from build123d import *

# Parameters (mm, degrees)
SKETCH1_R           = 38.1
BOSS_EXTRUDE1_DEPTH = 50.8
SKETCH2_W           = 38.1
SKETCH2_H           = 12.7
SKETCH2_W_2         = 1.5875
SKETCH2_H_2         = 34.925
SKETCH4_R           = 6.35
BOSS_EXTRUDE2_DEPTH = 6.35
BOSS_EXTRUDE3_DEPTH = 9.525
FILLET1_R           = 2.54
SKETCH6_W           = 3.175
SKETCH6_H           = 12.7
CUT_EXTRUDE1_DEPTH  = 12.7
SHELL1_START        = 3.81
SHELL1_OUTLINE_R    = 22.86
SHELL1_OUTLINE_W    = 8.255
SHELL1_OUTLINE_H    = 17.78
SHELL1_DEPTH        = 42.8625
SHELL1_START_2      = 7.9375
SHELL1_2_OUTLINE_W  = 8.255
SHELL1_2_OUTLINE_H  = 17.78
SHELL1_2_DEPTH      = 38.735
SHELL1_START_3      = 58.1025
SHELL1_3_DEPTH      = 4.445
SHELL1_START_4      = 46.6725
SHELL1_4_OUTLINE_R  = 3.81
SHELL1_4_DEPTH      = 11.43
SHELL1_START_5      = -2.2225
SHELL1_6_OUTLINE_R  = 19.05
SHELL1_6_OUTLINE_W  = 8.255
SHELL1_6_OUTLINE_H  = 17.78
SHELL1_6_DEPTH      = 6.0325


with BuildPart() as part:
    # Sketch1 → Boss-Extrude1 (new body)
    with BuildSketch(Plane.XY):
        Circle(SKETCH1_R)
    extrude(amount=BOSS_EXTRUDE1_DEPTH)

    # Sketch2 → Cut-Revolve1 (revolve, cut)
    with BuildSketch(Plane(origin=(0, 0, 0), x_dir=(0, 0, -1), z_dir=(1, 0, 0))):
        with Locations((-25.4, 31.75)):
            Rectangle(SKETCH2_W, SKETCH2_H)
        with Locations((-0.79375, 17.4625)):
            Rectangle(SKETCH2_W_2, SKETCH2_H_2)
        with Locations((-50.00625, 17.4625)):
            Rectangle(SKETCH2_W_2, SKETCH2_H_2)
    revolve(axis=Axis((0, 0, 0), (0, 0, 1)), mode=Mode.SUBTRACT)

    # Sketch3 → Revolve1 (revolve)
    with BuildSketch(Plane(origin=(0, 0, 0), x_dir=(0, 0, -1), z_dir=(1, 0, 0))):
        with BuildLine():
            Line((4.7625, 19.05), (4.7625, 0))
            Line((4.7625, 0), (-1.5875, 0))
            Line((-1.5875, 0), (-1.5875, 25.4))
            Line((-1.5875, 25.4), (1.99026356, 23.575552712))
            ThreePointArc((1.99026356, 23.575552712), (4.014349425, 21.703578821), (4.7625, 19.05))
        make_face()
    revolve(axis=Axis((0, 0, -4.7625), (0, 0, 1)))

    # Sketch4 → Boss-Extrude2 (add)
    with BuildSketch(Plane.XY.offset(49.2125)):
        with Locations(Location((0, 0, 0), (0, 0, 90))):
            Circle(SKETCH4_R)
    extrude(amount=BOSS_EXTRUDE2_DEPTH)

    # Sketch5 → Boss-Extrude3 (add)
    with BuildSketch(Plane.XY.offset(55.5625)):
        with BuildLine():
            Line((-2.358330795, 25.854173013), (-11.945334146, 1.886664636))
            ThreePointArc((-11.945334146, 1.886664636), (-12.308672556, 0), (-11.945334146, -1.886664636))
            Line((-11.945334146, -1.886664636), (-2.358330795, -25.854173013))
            ThreePointArc((-2.358330795, -25.854173013), (0, -27.450840695), (2.358330795, -25.854173013))
            Line((2.358330795, -25.854173013), (11.945334146, -1.886664636))
            ThreePointArc((11.945334146, -1.886664636), (12.308672556, 0), (11.945334146, 1.886664636))
            Line((11.945334146, 1.886664636), (2.358330795, 25.854173013))
            ThreePointArc((2.358330795, 25.854173013), (0, 27.450840695), (-2.358330795, 25.854173013))
        make_face()
    extrude(amount=BOSS_EXTRUDE3_DEPTH)

    # Fillet1
    fillet1_edges = [part.edges().sort_by_distance(p)[0] for p in [
        (0, -27.450840695, 65.0875),
        (7.15183247, -13.870418824, 65.0875),
        (12.308672556, 0, 65.0875),
        (7.15183247, 13.870418824, 65.0875),
        (0, 27.450840695, 65.0875),
        (-7.15183247, 13.870418824, 65.0875),
        (-12.308672556, 0, 65.0875),
        (-7.15183247, -13.870418824, 65.0875),
    ]]
    fillet(fillet1_edges, radius=FILLET1_R)

    # Sketch6 → Cut-Extrude1 (cut)
    with BuildSketch(Plane(origin=(0, 0, -4.7625), x_dir=(-1, 0, 0), z_dir=(0, 0, -1))):
        Rectangle(SKETCH6_W, SKETCH6_H)
    extrude(amount=-CUT_EXTRUDE1_DEPTH, mode=Mode.SUBTRACT)

    # Shell1: read off the stored shape, not the designer's step
    # Shell1 outline → Shell1 (cut)
    with BuildSketch(Plane.XY.offset(SHELL1_START)):
        Circle(SHELL1_OUTLINE_R)
        Rectangle(SHELL1_OUTLINE_W, SHELL1_OUTLINE_H, mode=Mode.SUBTRACT)
    extrude(amount=SHELL1_DEPTH, mode=Mode.SUBTRACT)

    # Shell1 2 outline → Shell1 2 (cut)
    with BuildSketch(Plane.XY.offset(SHELL1_START_2)):
        Rectangle(SHELL1_2_OUTLINE_W, SHELL1_2_OUTLINE_H)
    extrude(amount=SHELL1_2_DEPTH, mode=Mode.SUBTRACT)

    # Shell1 3 outline → Shell1 3 (cut)
    with BuildSketch(Plane.XY.offset(SHELL1_START_3)):
        with BuildLine():
            Line((9.587003351, 0.943332318), (0, 24.910840695))
            Line((0, 24.910840695), (-9.587003351, 0.943332318))
            ThreePointArc((-9.587003351, 0.943332318), (-9.768672556, 0), (-9.587003351, -0.943332318))
            Line((-9.587003351, -0.943332318), (0, -24.910840695))
            Line((0, -24.910840695), (9.587003351, -0.943332318))
            ThreePointArc((9.587003351, -0.943332318), (9.768672556, 0), (9.587003351, 0.943332318))
        make_face()
    extrude(amount=SHELL1_3_DEPTH, mode=Mode.SUBTRACT)

    # Shell1 4 outline → Shell1 4 (cut)
    with BuildSketch(Plane.XY.offset(SHELL1_START_4)):
        Circle(SHELL1_4_OUTLINE_R)
    extrude(amount=SHELL1_4_DEPTH, mode=Mode.SUBTRACT)

    # Shell1 5 outline → Shell1 5 (revolve, cut)
    with BuildSketch(Plane.XZ):
        with BuildLine():
            ThreePointArc((19.05, -2.2225), (20.37678941, -1.848424713), (21.312776356, -0.83638178))
            Line((21.312776356, -0.83638178), (23.682155577, 3.81))
            Line((23.682155577, 3.81), (19.05, 3.81))
            Line((19.05, 3.81), (19.05, -2.2225))
        make_face()
    revolve(axis=Axis((0, 0, 0), (0, 0, 1)), mode=Mode.SUBTRACT)

    # Shell1 6 outline → Shell1 6 (cut)
    with BuildSketch(Plane.XY.offset(SHELL1_START_5)):
        Circle(SHELL1_6_OUTLINE_R)
        Rectangle(SHELL1_6_OUTLINE_W, SHELL1_6_OUTLINE_H, mode=Mode.SUBTRACT)
    extrude(amount=SHELL1_6_DEPTH, mode=Mode.SUBTRACT)


solid = part.part
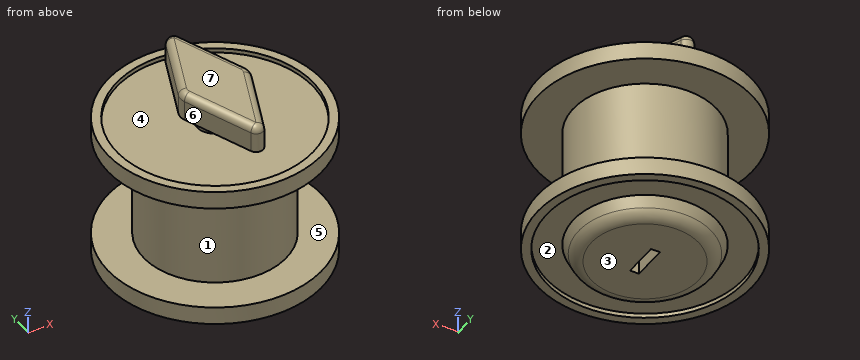
Read the model definition and answer for the solid it produces. Units are mm, in the model's axes. Face numbers are marked on the shaded views. A direction names the side the tool comes from. Coordinates: 2 decimals unless noted, no trailing zeros. Order: outer loops, then holes, each group sorted by start corner. A loop starts at its lowest first (then second) coordinate and runs counter-clockwise, first axis right, second up. Notation, with made-up numbers: (86, 11.5) -> (90, 11.5) arc R27 cw to (90, 36.5) -> close; hole circle Ø4 at (0, -39.75). An arc over 180 degrees is marked (long way). Answer as a JSON object with one key per item and string values.
1) A cutting plane is placed at C-C, the plane z = 23.5. Determine the outline of the cut face in (x, y), plus the area to 3 significant figures.
Model answer:
{"outline": "circle Ø50.8 at (0, 0); hole circle Ø45.72 at (0, 0)", "area": "385 mm²"}
2) Consider line 1 along Z through (x, y) = (5.5, -4.5); line 2 along Z through (x, y) = (-34, 10); line 3 along Z through (x, y) = (18, 2). Determine where each line is inside the solid, lowest interval first. Write a range as from..to.
Model answer:
{"line 1": "z = -4.76..-2.22, 46.67..49.21, 55.56..58.1, 62.55..65.09", "line 2": "z = 0..6.35, 44.45..50.8", "line 3": "z = -4.76..-2.22, 46.67..49.21"}
3) A cutting plane is placed at A-A, the plane y = -33. Determine the outline of the cut face in (x, z), plus the area to 3 significant figures.
Model answer:
{"outline": "(-19.04, 0) -> (-11.43, 0) -> (-11.43, 1.59) -> (11.43, 1.59) -> (11.43, 0) -> (19.04, 0) -> (19.04, 6.35) -> (-19.04, 6.35) -> close; (-19.04, 44.45) -> (19.04, 44.45) -> (19.04, 50.8) -> (11.43, 50.8) -> (11.43, 49.21) -> (-11.43, 49.21) -> (-11.43, 50.8) -> (-19.04, 50.8) -> close", "area": "411 mm²"}
4) A cutting plane is placed at B-B, the plane x = -32. Determine the outline of the cut face in (y, z).
Model answer:
{"outline": "(-20.68, 0) -> (-13.99, 0) -> (-13.99, 1.59) -> (13.99, 1.59) -> (13.99, 0) -> (20.68, 0) -> (20.68, 6.35) -> (-20.68, 6.35) -> close; (-20.68, 44.45) -> (20.68, 44.45) -> (20.68, 50.8) -> (13.99, 50.8) -> (13.99, 49.21) -> (-13.99, 49.21) -> (-13.99, 50.8) -> (-20.68, 50.8) -> close"}
5) A cutting plane is placed at D-D, the plane y = 16. State how many separate pieces and enclosed holes the cut face has, plus the area to 3 significant figures.
Model answer:
{"separate pieces": "2", "enclosed holes": "2", "area": "905 mm²"}
6) Each of these flat-tipped pins is pushed along its axis until it touches: pin 1 (3 mm diameter, centred on x = -26.5, y = -12, fed in from +Z); pin 2 (9 mm diameter, centred on x = 0, z = 2, fed in from -Y); pin 3 (4 mm diameter, centred on x = -9, z = 57, fed in from +Y); pin 4 (3 mm diameter, centred on x = 28, z = 37.5, fed in from -Y). Where does it stop, or does it pass through?
Model answer:
{"pin 1": "stops at z = 49.21", "pin 2": "stops at y = -38.1", "pin 3": "stops at y = 14.25", "pin 4": "passes through"}
7) A tool of negligible diameter and unlimited length cuts with its end or side. For the marked faces 1, 2 and 3, from which of +Z, -Z, +X, -X, +Y, -Y can it reach the whole face along a straight path? Write none if from no direction.
Model answer:
{"face 1": "none", "face 2": "-Z", "face 3": "-Z, +X, -X, +Y, -Y"}
8) The mould has two halves that part along Z. Classify the marked faces 4, 5, 6 and 7: released by +Z, released by -Z, zero draft, split by the parting line, or undercut.
Model answer:
{"face 4": "undercut", "face 5": "undercut", "face 6": "zero draft", "face 7": "released by +Z"}
